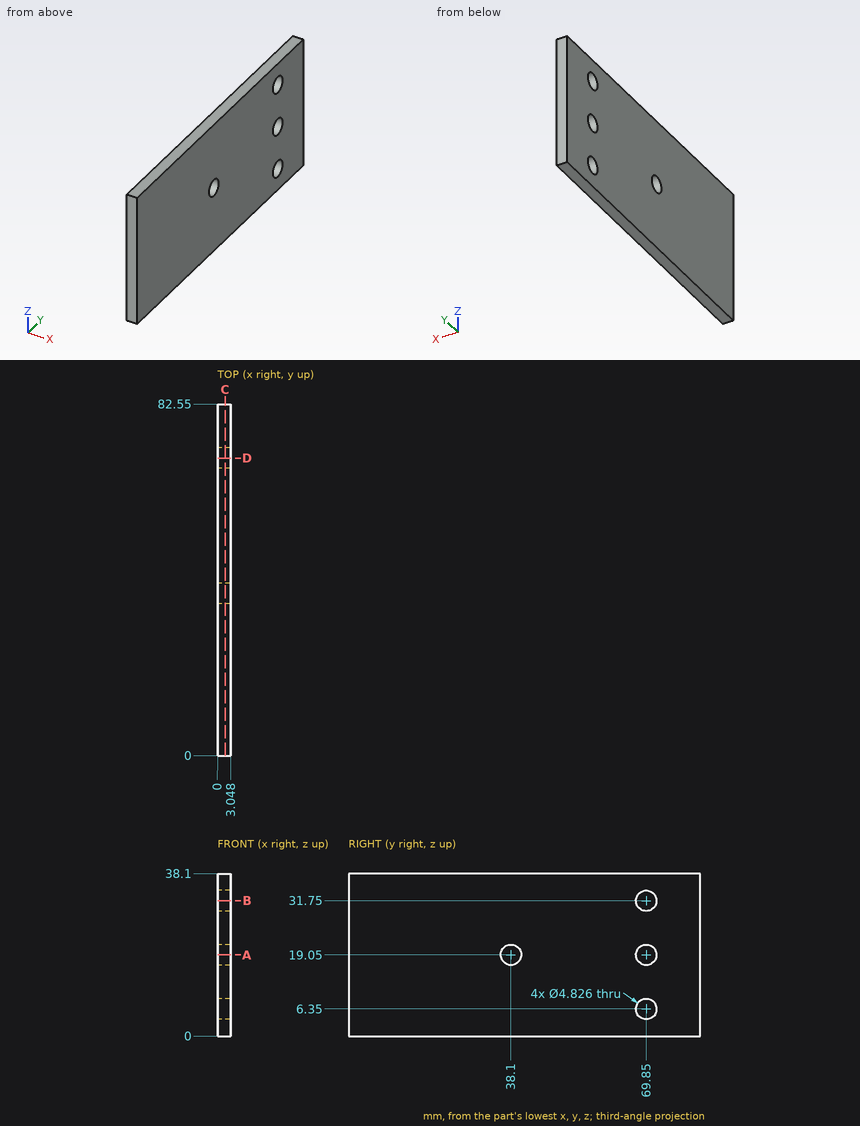
Can you work these out from the drawing? Everything is in mm from the part's minimum corner. Coordinates: 2 decimals unless noted, no trailing zeros. Loops run counter-clockwise (first coordinate to the right, second up) from the corner with the lowest first, then second, coordinate; pieces in that order, holes last. Notation, with made-up numbers: M -39.75,82.5 L -34.75,82.5 A8 ccw -34.75,89.5 Z; hole C -34,48.25 d4. An arc over 180 degrees is marked long. Put each result on its own line as item: value. Start each with the question number.
(1) I need wall thicknesses on line 1 (Y direction, x = 1.7, z = 19.05); line 2 (Z direction, x = 2.35, y = 69.85); line 3 (Y direction, x = 1, z = 6.35). Which ranges of each line are inside material? Lowest first, please. Write a range as from..to.
(2) Suppose I cut it at D-D on y = 69.85. Please give me the cut outline in (x, z).
(3) Suppose I cut it at A-A on z = 19.05. Please give me the cut outline in (x, y), then the cut area to 3 significant figures.
(4) Suppose I cut it at B-B on z = 31.75. Please give me the cut outline in (x, y), then the cut area to 3 significant figures.
(5) Suppose I cut it at C-C on x = 1.75. Please give me the cut outline in (y, z).
Solutions:
1. line 1: y = 0..35.69, 40.51..67.44, 72.26..82.55
1. line 2: z = 0..3.94, 8.76..16.64, 21.46..29.34, 34.16..38.1
1. line 3: y = 0..67.44, 72.26..82.55
2. outline: M 0,0 L 3.05,0 L 3.05,3.94 L 0,3.94 Z; M 0,8.76 L 3.05,8.76 L 3.05,16.64 L 0,16.64 Z; M 0,21.46 L 3.05,21.46 L 3.05,29.34 L 0,29.34 Z; M 0,34.16 L 3.05,34.16 L 3.05,38.1 L 0,38.1 Z
3. outline: M 0,0 L 3.05,0 L 3.05,35.69 L 0,35.69 Z; M 0,40.51 L 3.05,40.51 L 3.05,67.44 L 0,67.44 Z; M 0,72.26 L 3.05,72.26 L 3.05,82.55 L 0,82.55 Z
3. area: 222 mm2
4. outline: M 0,0 L 3.05,0 L 3.05,67.44 L 0,67.44 Z; M 0,72.26 L 3.05,72.26 L 3.05,82.55 L 0,82.55 Z
4. area: 237 mm2
5. outline: M 0,0 L 82.55,0 L 82.55,38.1 L 0,38.1 Z; hole C 38.1,19.05 d4.83; hole C 69.85,6.35 d4.83; hole C 69.85,19.05 d4.83; hole C 69.85,31.75 d4.83
